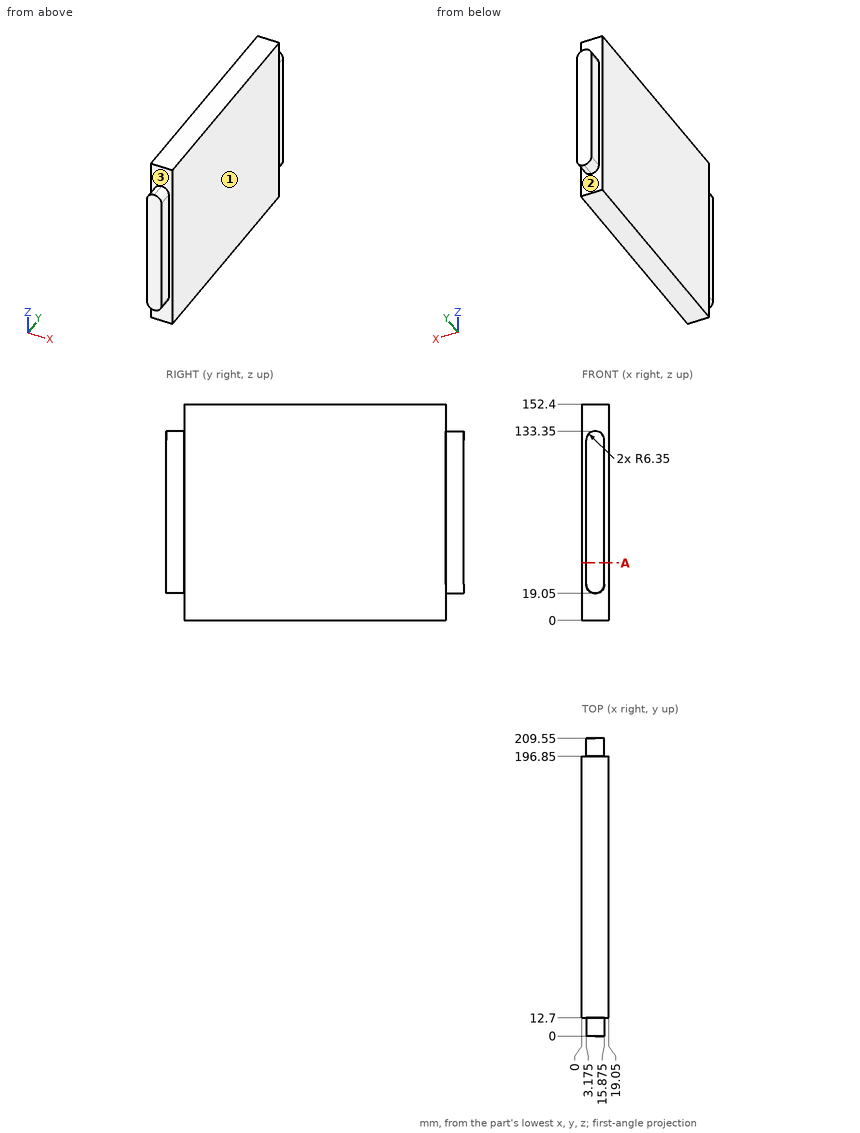
Geometry: see drawing. Coordinates: mm, zero at the bounding-box minimum. A direction names the side the tool comes from. Coordinates: 2 decimals unless noted, no trailing zeros. Loops run counter-clockwise (first coordinate to the right, second up) from the corner with the lowest first, then second, coordinate; pieces in that order, holes last. Notation, with made-up numbers: (79.5, 40) - (85.5, 40) arc R15 ccw to (85.5, 54) - close; hole circle Ø7 at (-40, 9.25). An arc over 180 degrees is marked (long way). Return JSON: item names as keys, results as strings.
Q1. Access query for the marked faces 1, 2 and 3. Directions: +Z, -Z, +X, -X, +Y, -Y. A direction counts if a zero-diameter tool reaches every point of the face in a straight line with its end or side. Return the directions, or none.
Results:
{"face 1": "+Z, -Z, +X, +Y, -Y", "face 2": "-X, +Y", "face 3": "-Y"}
Q2. Contact query for flat-ended pins moving along their axis: P1, Ø1, axis at x = 2.5, z = 21.5, coming from the -Y side; P2, Ø10, axis at y = 5.5, z = 70.5, coming from the +X side (3 decimals); P3, Ø6.5, axis at y = 6.5, z = 78, coming from the -X side (3 decimals). Output: stop coordinate, or through.
Results:
{"P1": "y = 12.7", "P2": "x = 15.875", "P3": "x = 3.175"}
Q3. Material intervals for line 1 along Y through (x, z) = (16, 112); line 2 along X through (y, z) = (200.5, 20.5), sorted ascending.
Results:
{"line 1": "12.7 to 196.85", "line 2": "5.49 to 13.56"}
Q4. Section A-A, the plane z = 40.5. Return loops of the section in (x, y) (3 decimals).
Results:
{"outline": "(0, 12.7) - (3.175, 12.7) - (3.175, 0) - (15.875, 0) - (15.875, 12.7) - (19.05, 12.7) - (19.05, 196.85) - (15.875, 196.85) - (15.875, 209.55) - (3.175, 209.55) - (3.175, 196.85) - (0, 196.85) - close"}
